Read the model definition and answer for the solid it produces. Units are mm, in the model's axes. A direction names the side the tool comes from. Round coordinates to 2 decimals unless told otherwise and drop trailing zeros. Loops run counter-clockwise (first coordinate to the right, second up) from the corner with the lowest first, then second, coordinate; pieces in that order, holes last. Notation, with made-up numbers: M 18.25,-16 L 34.25,-16 A15 cw 34.25,13 Z; hole C 35,-13 d8. An arc over 180 degrees is marked long. Write each question's results on one line, items separated by ' | '.
Autodesk Inventor part; units mm, degrees
ref_plane "YZ Plane" through (0, 0, 0) normal (1, 0, 0) x (0, 1, 0)
ref_plane "XZ Plane" through (0, 0, 0) normal (0, 1, 0) x (-1, 0, 0)
ref_plane "XY Plane" through (0, 0, 0) normal (0, 0, 1) x (1, 0, 0)
sketch "スケッチ1" plane through (0, 0, 0) normal (0, 1, 0) x (-1, 0, 0)
  circle A0 centre (0, 0) radius 7.5
  circle A1 centre (0, 0) radius 4.25
  circle A2 centre (0, 0) radius 1.5
  line L0 (0, 0) -> (0, 24)
  circle A3 centre (0, 24) radius 3.8
  line L1 (3.8, 24) -> (3.8, 12.8013)
  line L2 (-3.8, 24) -> (-3.8, 12.8013)
  circle A4 centre (0, 24) radius 1.5
  circle A5 centre (0, 19.5) radius 1.5
  circle A6 centre (0, 8.5) radius 1.5
  arc A7 (3.8, 12.8013) -> (6.6601, 3.4487) centre (30.7804, 15.9384) ccw
  arc A8 (-6.6601, 3.4487) -> (-3.8, 12.8013) centre (-30.7804, 15.9384) ccw
  line L3 (-3, 19.487) -> (3, 19.487)
  line L4 (3, 19.487) -> (3, 24.0195)
  line L5 (3, 24.0195) -> (-3, 24.0195)
  line L6 (-3, 24.0195) -> (-3, 19.487)
  circle A9 centre (0, 19.487) radius 3
  circle A10 centre (0, 24.0195) radius 3
  point P0 (3.8, 8)
  point P1 (-3.8, 8)
  point P2 (-6.6601, 3.4487)
  point P3 (3.8, 24)
  point P4 (-1.0476, 7.4265)
  point P5 (1.0476, 7.4265)
  dimension "d0" = 15
  dimension "d1" = 8.5
  dimension "d2" = 3
  dimension "d3" = 24
  dimension "d4" = 7.6
  dimension "d5" = 16
  dimension "d6" = 0
  dimension "d7" = 3
  dimension "d8" = 3
  dimension "d9" = 4.5
  dimension "d10" = 3
  dimension "d11" = 11
  dimension "d14" = 3
  dimension "d15" = 3
extrude "押し出し1" add sketch "スケッチ1" along normal blind 4 contours A0 A6 | A0 A6 L0 A9 L4 A3 L1 A7 | A8 L2 A3 L6 A9 L0 A6 A0 | A3 L4 A10 L6 | L4 A9 A3 | A3 A9 A10 L4 | A9 L3 A5 L0 | L0 A5 L3 A9 | L6 A10 A9 A3 | A3 A9 L6 | A9 L3 A5 A3 | A3 A5 L0 A10 A9 | A10 A9 L0 A4 L5 | L5 A4 A10 | A9 A3 A5 L3 | A9 A10 L0 A5 A3 | L5 A4 L0 A9 A10 | A10 L0 A9 | A9 L0 A10
extrude "押し出し2" add sketch "スケッチ1" against normal blind 2 contours L4 A9 A3 | A3 A9 A10 L4 | A9 L3 A5 L0 | L0 A5 L3 A9 | L6 A10 A9 A3 | A3 A9 L6 | A9 L3 A5 A3 | A3 A5 L0 A10 A9 | A10 A9 L0 A4 L5 | L5 A4 A10 | A9 A3 A5 L3 | A9 A10 L0 A5 A3 | L5 A4 L0 A9 A10 | A10 L0 A9 | A9 L0 A10
extrude "押し出し3" add sketch "スケッチ1" against normal blind 2 contours A0 A6
extrude "押し出し4" add sketch "スケッチ1" along normal blind 3 contours A1
properties part number "ServoMotor_Hone2" material "鋼、高強度、低合金"
1. Find section C-C, the plane y = -1.5. Give the vertices of the cut face in (x, z), then the cut area to 3 significant figures.
Completed:
outline: M -3,19.49 A3 ccw 3,19.49 L 3,24.02 A3 ccw -3,24.02 Z; M -1.05,7.43 A7.5 ccw long 1.05,7.43 A1.5 cw Z; hole C 0,0 d8.5; hole C 0,19.5 d3; hole C 0,24 d3 | area: 161 mm2
2. Determine the mould class of faces 1 (the face through (0.195, 0.958, 22.513)), 2 (the face through (-3.8, 2, 18)), 3 (the face through (4.786, 1.972, 8.061)) for opening direction X: released by +X, released by -X, zero draft, split by the parting line, or undercut.
Completed:
face 1: undercut | face 2: released by -X | face 3: released by +X
3. Find section A-A, the plane z = 0. Give the vertices of the cut face in (x, y), then the cut area to 3 significant figures.
Completed:
outline: M -7.5,-2 L -4.25,-2 L -4.25,0 L -1.5,0 L -1.5,3 L -4.25,3 L -4.25,4 L -7.5,4 Z; M 1.5,0 L 4.25,0 L 4.25,-2 L 7.5,-2 L 7.5,4 L 4.25,4 L 4.25,3 L 1.5,3 Z | area: 55.5 mm2
4. Find section D-D, the plane y = 1.45. Give the vertices of the cut face in (x, z).
Completed:
outline: M -6.66,3.45 A7.5 ccw long 6.66,3.45 A27.16 cw 3.8,12.8 L 3.8,24 A3.8 ccw -3.8,24 L -3.8,12.8 A27.16 cw Z; hole C 0,0 d3; hole C 0,8.5 d3; hole C 0,19.5 d3; hole C 0,24 d3
5. Given P1, Ø2, axis at y = 1.5, z = 23, coming from the -X side; P2, Ø1.5, axis at x = -1, z = -0.5, coming from the +Y side; P3, Ø0.6, axis at y = -1.5, z = 22, coming from the -X side; P4, Ø4, axis at x = 1.5, z = -2, coming from the +Y side, each flat-ended and moving along its own axis, determine where each tip first touches the part or whether it passes through.
Completed:
P1: stops at x = -3.8 | P2: stops at y = 3 | P3: stops at x = -3 | P4: stops at y = 4
6. Which of the six approach directions +Z, -Z, +X, -X, +Y, -Y give full straight-line access (tool end or side, diameter ignored) to faces 4 (the face through (-0.07, -0.99, 27.02)), 5 (the face through (-2, 0, 0)), 6 (the face through (3, -1, 22))?
Completed:
face 4: +Z, -Y | face 5: -Y | face 6: +Z, +X, -Y
7. Find section B-B, the plane x = 0. Count the separate pieces of the cut face and the enclosed holes in it, then the cut area to 3 significant figures.
Completed:
separate pieces: 5 | enclosed holes: 0 | area: 109 mm2
8. Find the intervals of material crossed by L1, parallel to Z at x = 0, y = 0.85; L2, parallel to Z at x = 0, y = -0.4; L3, parallel to X at y = 2.3, z = 0, in increasing order.
Completed:
L1: z = -7.5 to -1.5, 1.5 to 7, 10 to 18, 21 to 22.5, 25.5 to 27.8 | L2: z = -7.5 to -4.25, 4.25 to 7, 16.49 to 18, 21 to 22.5, 25.5 to 27.02 | L3: x = -7.5 to -1.5, 1.5 to 7.5
